Here's the drawing with two shaded views (mm, measured from the low corner). I have some questions. A direction names the side the tool comes from. Give positions to 0.01 mm unless a question says otherwise; leave off trailing zeros. Order: outer loops, then holes, each group sorted by start corner. A loop starts at its lowest first (then second) coordinate and runs counter-clockwise, first axis right, second up. Notation, with made-up numbers: M -8.75,22.5 L 5.25,22.5 A33 cw 5.25,51.5 Z; hole C 39.25,-27 d5. An arc over 180 degrees is marked long. Use a Markdown table: item, result. Add a question column.
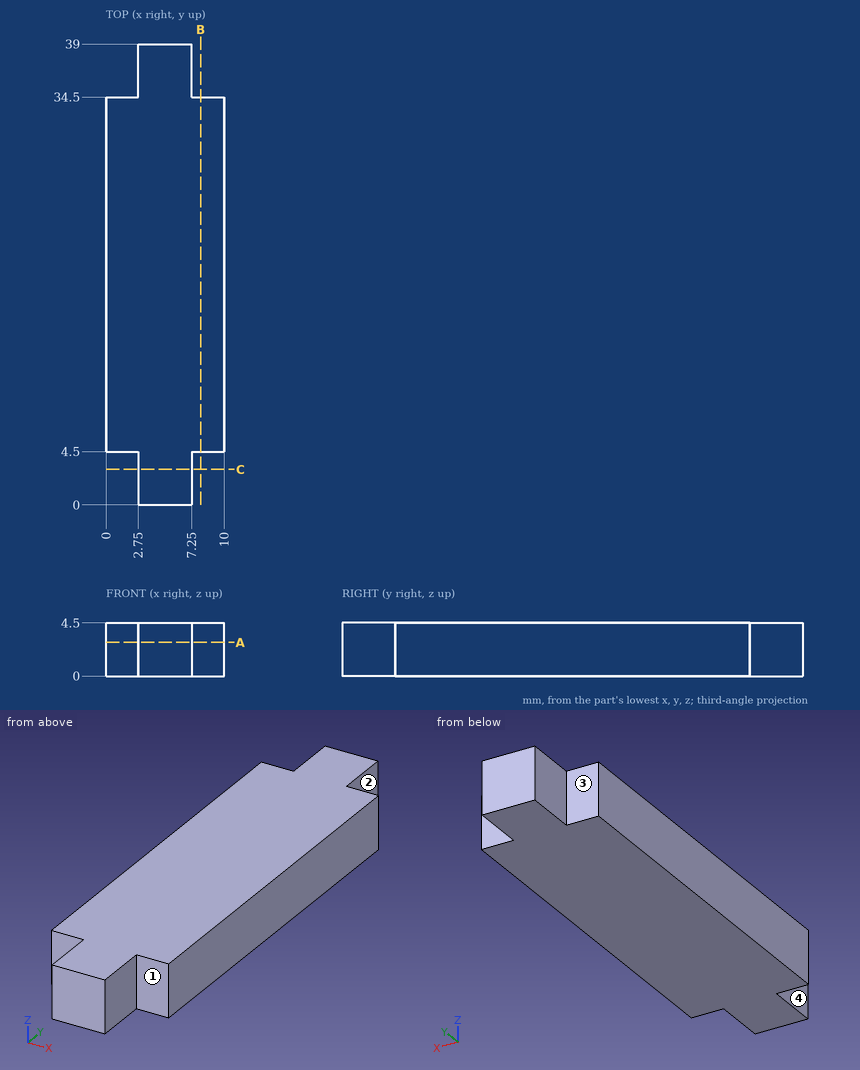
1) Suppose I cut it at B-B on x = 8. Please give me the cut outline in (y, z), and give its area (3 significant figures).
2) Suppose I cut it at A-A on z = 2.85. Please give me the cut outline in (x, y).
3) Please list where these lines run through material, in increasing order: line 1 (Y direction, x = 9.25, z = 2.1); line 2 (X direction, y = 35, z = 2.4). Write a range as from..to.
4) For the marked faces 1, 2, 3 and 4, which set-ups out of +Z, -Z, +X, -X, +Y, -Y let a thin tool reach every point of the face, with its end or its side?
5) Suppose I cut it at C-C on y = 3. Please give me the cut outline in (x, z), and give its area (4 significant figures).
6) For pin 1 (1.4 mm diameter, centred on x = 8, z = 2, fed in from +Y); pin 2 (1.3 mm diameter, centred on y = 36, z = 1, fed in from +X); pin 3 (1.3 mm diameter, centred on y = 1.5, z = 2, fed in from -X); pin 4 (4 mm diameter, centred on x = 3.5, y = 31.5, fed in from -Z), each with a flat end and sliding along its axis, tell me the tip position at first contact or that it passes through.
Values found:
| question | item | result |
|---|---|---|
| 1 | outline | M 4.5,0 L 34.5,0 L 34.5,4.5 L 4.5,4.5 Z |
| 1 | area | 135 mm^2 |
| 2 | outline | M 0,4.5 L 2.75,4.5 L 2.75,0 L 7.25,0 L 7.25,4.5 L 10,4.5 L 10,34.5 L 7.25,34.5 L 7.25,39 L 2.75,39 L 2.75,34.5 L 0,34.5 Z |
| 3 | line 1 | y = 4.5..34.5 |
| 3 | line 2 | x = 2.75..7.25 |
| 4 | face 1 | +Z, -Z, +X, -Y |
| 4 | face 2 | +Z, -Z, +X, +Y |
| 4 | face 3 | +Z, -Z, -X, +Y |
| 4 | face 4 | +Z, -Z, -X, -Y |
| 5 | outline | M 2.75,0 L 7.25,0 L 7.25,4.5 L 2.75,4.5 Z |
| 5 | area | 20.25 mm^2 |
| 6 | pin 1 | stops at y = 34.5 |
| 6 | pin 2 | stops at x = 7.25 |
| 6 | pin 3 | stops at x = 2.75 |
| 6 | pin 4 | stops at z = 0 |
